Design review of the part built by this model. Coordinates are the model's own, in mm. A direction names the side the tool comes from. Give positions to 0.01 mm unless a question says otherwise; leave off trailing zeros. Loops run counter-clockwise (first coordinate to the right, second up) from the corner with the lowest first, then second, coordinate; pieces in that order, holes last. Notation, with made-up numbers: (25.25, 60) - (60.25, 60) arc R26 ccw to (60.25, 85) - close; hole circle Ø9 at (-32.5, 54.25). An arc over 180 degrees is marked (long way). Put each result on its own line as item: value. Start each with the question number.
```python
from build123d import *

# Parameters (mm, degrees)
F0_R      = 100
F1_DEPTH  = 80
F3_DEPTH  = 80.001
F4_W      = 150.365841
F4_H      = 83.414628
F5_DEPTH  = 80.001
F6_R      = 7.5
F6_R_2    = 70
F7_DEPTH  = 20
F9_DEPTH  = 25.001
F10_W     = 20
F10_H     = 15
F11_DEPTH = 10


with BuildPart() as f1:
    # F0 (on Front) → F1 (new body)
    with BuildSketch(Plane.XZ):
        Circle(F0_R)
    extrude(amount=-F1_DEPTH)

    # F2 (on face) → F3 (cut, through all)
    with BuildSketch(Plane.XZ):
        with BuildLine():
            Line((0, 0), (0, 100))
            ThreePointArc((0, 100), (-70.710678, -70.710678), (100, 0))
            Line((100, 0), (0, 0))
        make_face()
    extrude(amount=-F3_DEPTH, mode=Mode.SUBTRACT)

    # F4 (on face) → F5 (cut, through all)
    with BuildSketch(Plane.XZ):
        with Locations((51.838493, 86.707314)):
            Rectangle(F4_W, F4_H)
    extrude(amount=-F5_DEPTH, mode=Mode.SUBTRACT)

    # F6 (on face) → F7 (cut)
    with BuildSketch(Plane.XY.offset(45)):
        with Locations((60, 65)):
            Circle(F6_R)
        Circle(F6_R_2)
    extrude(amount=-F7_DEPTH, mode=Mode.SUBTRACT)

    # F8 (on face) → F9 (cut, through all)
    with BuildSketch(Plane.XY.offset(25)):
        with BuildLine():
            ThreePointArc((63.245553, 30), (51.453576, 47.460821), (35, 60.621778))
            Line((35, 60.621778), (35, 30))
            Line((35, 30), (63.245553, 30))
        make_face()
    extrude(amount=-F9_DEPTH, mode=Mode.SUBTRACT)

    # F10 (on face) → F11 (join)
    with BuildSketch(Plane.XY.offset(25)):
        with Locations((10, 7.5)):
            Rectangle(F10_W, F10_H)
    extrude(amount=F11_DEPTH)


solid = f1.part
```
Item 1: Mouldability with a two-part tool opening along X and no side actions: class faces 1 (the flat face through (0, 39, 17)), 2 (the flat face through (35, 46, 13)), 3 (the cylindrical face through (97.364, 39.44, 22.809)), 4 (the flat face through (10, 15, 30)) as pulls with the +X half, pulls with the -X half, needs draft (parallel to the pull), parting line crosses it, or undercut.
Item 2: For L1, parallel to Z at x = 37.5, y = 16; L2, parallel to X at y = 48, z = 3; L3, parallel to Y at x = 60, z = 29, list the stretches that pass through material, from the lowest coordinate up. Write a range as from..to.
Item 3: For P1, Ø8, axis at y = 49.5, z = 18.5, coming from the +X side; P2, Ø11, axis at y = 5, z = 27.5, coming from the +X side; P3, Ø12, axis at x = 45, y = 68, coming from the -Z side; P4, Ø7.5, axis at x = 12.5, y = 4, coming from the +Z side, all flat-tipped, find the tip position at first contact; note any pin that passes through.
Item 4: Consider section A-A (z = 32). State the section outline as (x, y) points, plus the area to 3 significant figures.
Item 5: Consider section D-D (z = 23.5). State the section outline as (x, y) points.
Item 6: Consider section C-C (y = 34). State the section outline as (x, z) points, plus the area to 3 significant figures.
Item 7: Machinability: for faces 5 (the flat face through (10, 8, 35)), 6 (the flat face through (49, 30, 13)), 7 (the flat face through (62, 39, 0)), 8 (the flat face through (20, 7, 30)), 9 (the cylindrical face through (54.5, 70.1, 35.1)), which of the approach directions +Z, -Z, +X, -X, +Y, -Y give a long, thin tool a straight path to every point of the face, cutting with its end or side? Answer none if there is none.
Item 8: Consider section B-B (x = 60). State the section outline as (y, z) points.
Geometry says:
1. face 1: pulls with the -X half
1. face 2: undercut
1. face 3: pulls with the +X half
1. face 4: needs draft
2. L1: z = 0..25
2. L2: x = 0..35, 50.95..99.95
2. L3: y = 36.06..57.5, 72.5..80
3. P1: stops at x = 98.94
3. P2: stops at x = 97.55
3. P3: stops at z = 0
3. P4: stops at z = 35
4. outline: (0, 0) - (20, 0) - (20, 15) - (0, 15) - close; (0, 70) arc R70 cw to (70, 0) - (94.74, 0) - (94.74, 80) - (0, 80) - close; hole circle Ø15 at (60, 65)
4. area: 3,850 mm2
5. outline: (0, 0) - (97.2, 0) - (97.2, 80) - (0, 80) - close; hole (35, 30) - (63.25, 30) arc R70 ccw to (35, 60.62) - close
6. outline: (0, 0) - (35, 0) - (35, 25) - (0, 25) - close; (61.19, 0) - (100, 0) arc R100 ccw to (89.3, 45) - (61.19, 45) - close
6. area: 2,460 mm2
7. face 5: +Z, -X, -Y
7. face 6: +Z, -Z
7. face 7: -Z, +X, -X, +Y, -Y
7. face 8: +Z, -Y
7. face 9: +Z
8. outline: (0, 0) - (30, 0) - (30, 25) - (0, 25) - close; (36.06, 0) - (80, 0) - (80, 45) - (72.5, 45) - (72.5, 25) - (57.5, 25) - (57.5, 45) - (36.06, 45) - close
